CAD build for the part. Positions are in the model's coordinates, mm. A direction names the side the tool comes from. Give positions to 0.01 mm unless a question says otherwise; leave off trailing zeros. Write each loop counter-clockwise with the first axis right and the second up, starting at its lowest first coordinate (ties: lowest second). Pieces come first, ordered by that corner, then holes. Notation, with made-up numbers: M 36,35.5 L 81,35.5 A32 cw 81,69.5 Z; hole C -28.75,-33 d6. An arc over 180 degrees is marked long. One line per question, with ' | ' between items. Start each with the question number.
1. Cut at A-A, the plane y = -20. Write the cut outline in (x, z), then the cut area to 3 significant figures.
2. Pull direction Y, two halves, no side cores. Call faces 1 (the face through (1, -30, -1)), 2 (the face through (1, -17, 105)), 3 (the face through (1, -35, -1)): released by +Y, released by -Y, zero draft, split by the parting line, or undercut.
3. Flat gauge pins, fed straight in: pin 1 (3.5 mm diameter, centred on x = 7.5, z = 52.99, fed in from +Y); pin 2 (1.5 mm diameter, centred on x = -134.5, z = -161.5, fed in from -Y). Where does each tip first touch, or does it go through?
4. Wall check: L1, parallel to Y at x = 15, z = 57.5; L2, parallel to Z at x = -248, y = -27.5; L3, parallel to X at y = -32.55, z = 40. Give the ranges that are in metal, low to high.
5. Which spindle directions (+Z, -Z, +X, -X, +Y, -Y) get a long thin tool onto all of the face, cutting with end or side? Do faces 4 (the face through (275, -27, 4)), 5 (the face through (-280, 10, 4)), 6 (the face through (275, 38, 4)), 7 (the face through (280, 10, 4)), 8 (the face through (1, -15, -100)). Say none if no direction does.
```python
from build123d import *

# Parameters (mm, degrees)
SKETCH1_W           = 560
SKETCH1_H           = 560
BOSS_EXTRUDE1_DEPTH = 5
SKETCH2_W           = 560
SKETCH2_H           = 560
SKETCH2_W_2         = 550
SKETCH2_H_2         = 550
BOSS_EXTRUDE2_DEPTH = 65
BOSS_EXTRUDE3_START = -5
SKETCH2_2_W         = 560
SKETCH2_2_H         = 560
SKETCH2_2_W_2       = 550
SKETCH2_2_H_2       = 550
BOSS_EXTRUDE3_DEPTH = 50
SKETCH7_W           = 100
SKETCH7_H           = 200
BOSS_EXTRUDE5_DEPTH = 5
SKETCH8_W           = 100
SKETCH8_H           = 35
BOSS_EXTRUDE6_DEPTH = 5
SKETCH9_R           = 3
CUT_EXTRUDE1_DEPTH  = 5
FILLET1_R           = 5
FILLET2_R           = 2.5
FILLET3_R           = 5


# Some blends are built 0.0001 mm under size
with BuildPart() as part:
    # Sketch1 → Boss-Extrude1 (new body)
    with BuildSketch(Plane(origin=(0, 0, 0), x_dir=(1, 0, 0), z_dir=(0, 1, 0))):
        Rectangle(SKETCH1_W, SKETCH1_H)
    extrude(amount=BOSS_EXTRUDE1_DEPTH)

    # Sketch2 → Boss-Extrude2 (add)
    with BuildSketch(Plane(origin=(0, 5, 0), x_dir=(1, 0, 0), z_dir=(0, 1, 0))):
        Rectangle(SKETCH2_W, SKETCH2_H)
        Rectangle(SKETCH2_W_2, SKETCH2_H_2, mode=Mode.SUBTRACT)
    extrude(amount=BOSS_EXTRUDE2_DEPTH)

    # Sketch2<2> → Boss-Extrude3 (add)
    with BuildSketch(Plane(origin=(0, 5, 0), x_dir=(1, 0, 0), z_dir=(0, 1, 0)).offset(BOSS_EXTRUDE3_START)):
        Rectangle(SKETCH2_2_W, SKETCH2_2_H)
        Rectangle(SKETCH2_2_W_2, SKETCH2_2_H_2, mode=Mode.SUBTRACT)
    extrude(amount=-BOSS_EXTRUDE3_DEPTH)



with BuildPart() as body_2:
    # Sketch7 → Boss-Extrude5 (new body)
    with BuildSketch(Plane(origin=(0, -30, 0), x_dir=(-1, 0, 0), z_dir=(0, -1, 0))):
        Rectangle(SKETCH7_W, SKETCH7_H)
    extrude(amount=BOSS_EXTRUDE5_DEPTH)


with BuildPart() as part_1:
    add(part.part)

    add(body_2.part)  # Boss-Extrude6 merges body 2
    # Sketch8 → Boss-Extrude6 (add)
    with BuildSketch(Plane(origin=(0, 0, -100), x_dir=(-1, 0, 0), z_dir=(0, 0, -1))):
        with Locations((0, -17.5)):
            Rectangle(SKETCH8_W, SKETCH8_H)
    boss_extrude6 = extrude(amount=BOSS_EXTRUDE6_DEPTH)

    # Mirror1: Boss-Extrude6 across plane
    add(boss_extrude6.mirror(Plane(origin=(0, 0, 0), x_dir=(1, 0, 0), z_dir=(0, 0, -1))))

    # Sketch9 → Cut-Extrude1 (cut)
    with BuildSketch(Plane.XZ.offset(35)):
        with Locations(Location((7.5, 52.990381057, 0), (0, 0, 270))):
            Circle(SKETCH9_R)
        with Locations(Location((0, 40, 0), (0, 0, 270))):
            Circle(SKETCH9_R)
        with Locations(Location((-7.5, 52.990381057, 0), (0, 0, 270))):
            Circle(SKETCH9_R)
    extrude(amount=-CUT_EXTRUDE1_DEPTH, mode=Mode.SUBTRACT)

    # Fillet1
    fillet1_edges = [part_1.edges().sort_by_distance(p)[0] for p in [
        (275, 5, 0),
        (0, 5, -275),
        (-275, 5, 0),
        (0, 5, 275),
        (275, 37.5, -275),
        (-275, 37.5, -275),
        (-275, 37.5, 275),
        (275, 37.5, 275),
        (275, 0, 0),
        (275, -25, 275),
        (0, 0, 275),
        (-275, -25, 275),
        (-275, 0, 0),
        (-275, -25, -275),
        (0, 0, -275),
        (275, -25, -275),
        (0, -35, -105),
        (0, 0, -105),
        (0, 0, 105),
        (0, -35, 105),
    ]]
    fillet(fillet1_edges, radius=FILLET1_R)

    # Fillet2
    fillet2_edges = [part_1.edges().sort_by_distance(p)[0] for p in [
        (275, 70, 0),
        (0, 70, -275),
        (0, 70, 275),
        (-275, 70, 0),
        (273.535533906, 70, -273.535533906),
        (273.535533906, 70, 273.535533906),
        (-273.535533906, 70, 273.535533906),
        (-273.535533906, 70, -273.535533906),
        (0, 70, 280),
        (280, 70, 0),
        (0, 70, -280),
        (-280, 70, 0),
    ]]
    fillet(fillet2_edges, radius=FILLET2_R - 0.0001)  # a hair under: the kernel refuses the full size

    # Fillet3
    # the kernel refuses this fillet: 5 mm, written as the material it takes off along each edge
    with BuildSketch(Plane(origin=(275, 70, 275), x_dir=(0, 0, 1), z_dir=(-1, 0, 0))) as fillet3_piece_1:
        with BuildLine():
            CenterArc((2.5001, -2.4999), 2.4999, 0, 90)
            Line((5, -2.4999), (5, 0))
            Line((5, 0), (2.5001, 0))
        make_face()
    revolve(axis=Axis((275, 70, 275), (0, 1, 0)), revolution_arc=90, mode=Mode.SUBTRACT)
    with BuildSketch(Plane(origin=(-275, 70, 275), x_dir=(-1, 0, 0), z_dir=(0, 0, -1))) as fillet3_piece_2:
        with BuildLine():
            CenterArc((2.5001, -2.4999), 2.4999, 0, 90)
            Line((5, -2.4999), (5, 0))
            Line((5, 0), (2.5001, 0))
        make_face()
    revolve(axis=Axis((-275, 70, 275), (0, 1, 0)), revolution_arc=90, mode=Mode.SUBTRACT)
    with BuildSketch(Plane(origin=(-275, 70, -275), x_dir=(0, 0, -1), z_dir=(1, 0, 0))) as fillet3_piece_3:
        with BuildLine():
            CenterArc((2.5001, -2.4999), 2.4999, 0, 90)
            Line((5, -2.4999), (5, 0))
            Line((5, 0), (2.5001, 0))
        make_face()
    revolve(axis=Axis((-275, 70, -275), (0, 1, 0)), revolution_arc=90, mode=Mode.SUBTRACT)
    with BuildSketch(Plane(origin=(275, 70, -275), x_dir=(1, 0, 0), z_dir=(0, 0, 1))) as fillet3_piece_4:
        with BuildLine():
            CenterArc((2.5001, -2.4999), 2.4999, 0, 90)
            Line((5, -2.4999), (5, 0))
            Line((5, 0), (2.5001, 0))
        make_face()
    revolve(axis=Axis((275, 70, -275), (0, 1, 0)), revolution_arc=90, mode=Mode.SUBTRACT)
    with BuildSketch(Plane(origin=(-280, -62.5, -280), x_dir=(0, 0, 1), z_dir=(0, 1, 0)), Plane(origin=(-280, -62.5, 280), x_dir=(1, 0, 0), z_dir=(0, 1, 0)), Plane(origin=(280, 70, -280), x_dir=(0, 0, 1), z_dir=(0, -1, 0)), Plane(origin=(280, 70, 280), x_dir=(-1, 0, 0), z_dir=(0, -1, 0))) as fillet3_piece_5:
        with BuildLine():
            CenterArc((FILLET3_R, FILLET3_R), FILLET3_R, 180, 90)
            Line((0, FILLET3_R), (0, 0))
            Line((0, 0), (FILLET3_R, 0))
        make_face()
    extrude(amount=132.5, mode=Mode.SUBTRACT)


solid = part_1.part
```
Here are the results:
1) outline: M -280,-275 A5 ccw -275,-280 L 275,-280 A5 ccw 280,-275 L 280,275 A5 ccw 275,280 L -275,280 A5 ccw -280,275 Z; M -50,-105 L 50,-105 L 50,-100 L -50,-100 Z; M -50,100 L 50,100 L 50,105 L -50,105 Z; hole M -275,-270 A5 ccw -270,-275 L 270,-275 A5 ccw 275,-270 L 275,270 A5 ccw 270,275 L -270,275 A5 ccw -275,270 Z | area: 12,100 mm^2
2) face 1: undercut | face 2: zero draft | face 3: released by -Y
3) pin 1: y = 5 | pin 2: y = 0
4) L1: -35 to -30, 0 to 5 | L2: -280 to -275, 275 to 280 | L3: -280 to -275, -50 to -3, 3 to 50, 275 to 280
5) face 4: -Y | face 5: +Z, -Z, -X, +Y, -Y | face 6: +Y | face 7: +Z, -Z, +X, +Y, -Y | face 8: none
